Autodesk Fusion 360 part; units mm, degrees
sketch "Sketch1" plane through (0, 0, 0) normal (0, 0, 1) x (1, 0, 0)
  line L0 (0, 0) -> (17.1, 0)
  line L1 (17.1, 0) -> (17.1, 2)
  line L2 (17.1, 2) -> (0, 2)
  line L3 (0, 2) -> (0, 0)
  line L4 (0, 0) -> (1.25, 0)
  line L5 (1.25, 0) -> (2.75, 0)
  circle A0 centre (2.75, 0) radius 1.5
  line L6 (4.25, 0) -> (7.05, 0)
  line L7 (7.05, 0) -> (8.55, 0)
  circle A1 centre (8.55, 0) radius 1.5
  line L8 (10.05, 0) -> (12.85, 0)
  line L9 (12.85, 0) -> (14.35, 0)
  circle A2 centre (14.35, 0) radius 1.5
  line L10 (15.85, 0) -> (17.1, 0)
  line L11 (15.85, 0) -> (17.4, 0)
  line L12 (17.4, 0) -> (18.95, 0)
  line L13 (18.95, 0) -> (17.1, 0)
  line L14 (17.1, 0) -> (17.1, 2)
  line L15 (17.1, 2) -> (18.95, 2)
  line L16 (18.95, 2) -> (18.95, 0)
  line L17 (17.1, 2) -> (34.2, 2)
  line L18 (34.2, 0) -> (17.1, 0)
  line L19 (18.95, 0) -> (20.45, 0)
  circle A3 centre (20.45, 0) radius 1.5
  line L20 (21.95, 0) -> (24.75, 0)
  line L21 (24.75, 0) -> (26.25, 0)
  circle A4 centre (26.25, 0) radius 1.5
  line L22 (27.75, 0) -> (30.55, 0)
  line L23 (30.55, 0) -> (32.05, 0)
  circle A5 centre (32.05, 0) radius 1.5
  line L24 (33.55, 0) -> (34.8, 0)
  line L25 (34.8, 0) -> (33.05, 0)
  line L26 (33.05, 0) -> (33.05, 2)
  line L27 (33.05, 2) -> (34.8, 2)
  line L28 (34.8, 2) -> (34.8, 0)
  dimension "d1" = 17.1
  dimension "d2" = 2
  dimension "d3" = 1.25
  dimension "d4" = 1.5
  dimension "d5" = 2.8
  dimension "d6" = 1.5
  dimension "d7" = 2.8
  dimension "d8" = 1.5
  dimension "d32" = 1.55
  dimension "d33" = 1.55
  dimension "d39" = 1.5
  dimension "d41" = 2.8
  dimension "d42" = 1.5
  dimension "d43" = 2.8
  dimension "d44" = 1.5
  dimension "d45" = 1.25
extrude "Extrude1" add sketch "Sketch1" along normal blind 10 contours L0 L1 L2 L3 L4 A0 L6 A1 L8 A2 L10 L11 L14 | L1 L11 L12 L13 L14 L15 L16 L17 L18 | L16 L17 L18 A3 L20 A4 L22 A5 L26 | L17 L18 A5 L24 L25 L26 L27 L28
sketch "Sketch10" plane through (0, 0, 0) normal (0, -1, 0) x (1, 0, 0)
  line L0 (15.85, 0) -> (18.95, 0)
  line L1 (18.95, 0) -> (18.95, 10)
  line L2 (18.95, 10) -> (15.85, 10)
  line L3 (15.85, 10) -> (15.85, 0)
  line L4 (15.85, 0) -> (18.95, 0)
  line L5 (17.4, 0) -> (17.4, 10)
  circle A0 centre (17.4, 5) radius 1.5
  dimension "d46" = 3
extrude "Extrude6" cut sketch "Sketch10" against normal blind 2.6 contours L5 A0 | L5 A0
sketch "Sketch7" plane through (0, 2, 0) normal (0, 1, 0) x (-1, 0, 0)
  line L0 (-34.8, 0) -> (0, 0)
  line L1 (0, 0) -> (0, 10)
  line L2 (0, 10) -> (-34.8, 10)
  line L3 (0, 0) -> (0, 10)
  line L4 (0, 0) -> (-34.8, 0)
  line L5 (-17.4, 0) -> (-17.4, 10)
  circle A0 centre (0, 5) radius 5
  line L6 (0, 5) -> (5, 5)
  circle A1 centre (-17.4, 5) radius 1.5
  line L7 (-34.8, 10) -> (-34.8, 0)
  line L8 (2.5, 5) -> (0, 5)
  line L9 (2.5, 5) -> (2.1, 5)
  line L10 (2.5, 5) -> (0.5, 5)
  line L11 (2.5, 5) -> (1, 5)
  line L12 (1, 5) -> (1.5, 5)
  circle A2 centre (1.5, 5) radius 1.5
  circle A3 centre (-34.8, 5) radius 5
  circle A4 centre (-36.3, 5) radius 1.5
  line L13 (0, 10) -> (-1.25, 10)
  line L14 (-1.25, 10) -> (-1.25, 0)
  line L15 (5, 5) -> (-1.25, 5)
  dimension "d49" = 0.4
  dimension "d50" = 2
  dimension "d52" = 0.5
extrude "Extrude5" add sketch "Sketch7" against normal blind 2 contours L7 A3 | L1 L3 A0 L6 A2 L15 | L1 L3 A0 L6 A2 L15 picked at (-35.3657, 1.2198)
Design review of the part built by this model. Coordinates are the model's own, in mm. Give positions to 0.01 mm unless a question says otherwise; leave off trailing zeros. Write each loop counter-clockwise with the first axis right and the second up, starting at its lowest first coordinate (ties: lowest second). Pieces come first, ordered by that corner, then holes.
(1) Add section A-A (x = 17.4). Give the boundary of the cut face in (y, z), and give its area (3 significant figures).
Checked values:
outline: (0, 0) - (2, 0) - (2, 3.5) - (0, 3.5) - close; (0, 6.5) - (2, 6.5) - (2, 10) - (0, 10) - close
area: 14.0 mm2
(2) Add section B-B (y = 1.1). Give the number of separate pieces and of enclosed holes in the cut face, and give its area (3 significant figures).
Checked values:
separate pieces: 7
enclosed holes: 3
area: 283 mm2
(3) Wall thickness on line 1 along Z through (x, y) = (36.3, 0.65); line 2 along Z through (x, y) = (36, 1.2); line 3 along Y through (x, z) = (13, 3.5): over which ranges is each line inside the solid? List them lowest first.
Checked values:
line 1: z = 0.23 to 3.5, 6.5 to 9.77
line 2: z = 0.15 to 3.53, 6.47 to 9.85
line 3: y = 0.65 to 2
(4) Add section C-C (z = 1). Give the boundary of the cut face in (x, y).
Checked values:
outline: (-3, 0) - (1.25, 0) arc R1.5 cw to (4.25, 0) - (7.05, 0) arc R1.5 cw to (10.05, 0) - (12.85, 0) arc R1.5 cw to (15.85, 0) - (18.95, 0) arc R1.5 cw to (21.95, 0) - (24.75, 0) arc R1.5 cw to (27.75, 0) - (30.55, 0) arc R1.5 cw to (33.55, 0) - (37.8, 0) - (37.8, 2) - (-3, 2) - close
(5) Clearance check with a flat-ended pin moving along its axis: pin 1 Ø5 at (x, z) = (17.4, 5) entering from +Y. State where the tip first meets the part, or that it passes through.
Checked values:
pin 1: stops at y = 2
(6) Add section D-D (z = 4.5). Give the boundary of the cut face in (x, y), and give its area (3 significant figures).
Checked values:
outline: (-4.97, 0) - (-2.91, 0) - (-2.91, 2) - (-4.97, 2) - close; (-0.09, 0) - (1.25, 0) arc R1.5 cw to (4.25, 0) - (7.05, 0) arc R1.5 cw to (10.05, 0) - (12.85, 0) arc R1.5 cw to (15.85, 0) - (15.99, 0) - (15.99, 2) - (-0.09, 2) - close; (18.81, 0) - (18.95, 0) arc R1.5 cw to (21.95, 0) - (24.75, 0) arc R1.5 cw to (27.75, 0) - (30.55, 0) arc R1.5 cw to (33.55, 0) - (34.89, 0) - (34.89, 2) - (18.81, 2) - close; (37.71, 0) - (39.77, 0) - (39.77, 2) - (37.71, 2) - close
area: 51.3 mm2
